CAD build for the part. Positions are in the model's coordinates, mm. Coordinates: 2 decimals unless noted, no trailing zeros. Write each loop counter-clockwise with the first axis right and the second up, starting at its lowest first coordinate (ties: lowest second). Pieces come first, ordered by that corner, then holes. Notation, with made-up numbers: M 58,5 L 70,5 A23 ccw 70,16 Z; hole C 12.5,48 d7. An arc over 180 degrees is marked long. Put each result on its own line as item: value. Start each with the question number.
```python
from build123d import *

# Parameters (mm, degrees)
SKETCH1_W           = 1346.2
SKETCH1_H           = 1143
BOSS_EXTRUDE1_DEPTH = 1.27
CUT_EXTRUDE1_DEPTH  = 3.54


with BuildPart() as part:
    # Sketch1 → Boss-Extrude1 (new body, symmetric)
    with BuildSketch(Plane.XY):
        Rectangle(SKETCH1_W, SKETCH1_H)
    extrude(amount=BOSS_EXTRUDE1_DEPTH, both=True)

    # Sketch2 → Cut-Extrude1 (cut, through all)
    with BuildSketch(Plane.XY.offset(1.27)):
        with BuildLine():
            Line((-673.1, 546.1), (-673.1, -546.1))
            add(Edge.make_bspline(
                [(-152.4, -224.495117073), (-152.4, -258.704669829), (-224.053162497, -532.777731838), (-673.1, -546.1)],
                knots=[0, 0, 0, 0, 1, 1, 1, 1], degree=3))
            Line((-152.4, -224.495117073), (-152.4, 224.495117073))
            add(Edge.make_bspline(
                [(-152.4, 224.495117073), (-152.4, 258.704669829), (-224.053162497, 532.777731838), (-673.1, 546.1)],
                knots=[0, 0, 0, 0, 1, 1, 1, 1], degree=3))
        make_face()
        with BuildLine():
            Line((673.1, 546.1), (673.1, -546.1))
            add(Edge.make_bspline(
                [(152.4, -224.495117073), (152.4, -258.704669829), (224.053162497, -532.777731838), (673.1, -546.1)],
                knots=[0, 0, 0, 0, 1, 1, 1, 1], degree=3))
            Line((152.4, -224.495117073), (152.4, 224.495117073))
            add(Edge.make_bspline(
                [(152.4, 224.495117073), (152.4, 258.704669829), (224.053162497, 532.777731838), (673.1, 546.1)],
                knots=[0, 0, 0, 0, 1, 1, 1, 1], degree=3))
        make_face()
    extrude(amount=-CUT_EXTRUDE1_DEPTH, mode=Mode.SUBTRACT)


solid = part.part
```
(1) Drop flat-ended pins along their axis: pin 1 (0.8 mm diameter, centred on y = -22, z = 0, fed in from +X); pin 2 (0.8 mm diameter, centred on y = 21, z = 0, fed in from -X). Give the stop position or say it passes through.
(2) Drill centre lines: line 1 (X direction, y = -119, z = 0.1); line 2 (Y direction, x = -465.5, z = -0.65); line 3 (Y direction, x = -456, z = 0). Where is each one in solid material? Low to high. Write a range as [from, to].
(3) Slice it at A-A, the plane y = 3.5. Write the cut outline in (x, z), then the cut area to 3 significant figures.
Result set:
1. pin 1: stops at x = 152.4
1. pin 2: stops at x = -152.4
2. line 1: x = [-152.4, 152.4]
2. line 2: y = [-571.5, -516.48], [516.48, 571.5]
2. line 3: y = [-571.5, -513.73], [513.73, 571.5]
3. outline: M -152.4,-1.27 L 152.4,-1.27 L 152.4,1.27 L -152.4,1.27 Z
3. area: 774 mm^2
